Autodesk Inventor part; units mm, degrees
ref_plane "Work Plane1" through (0, 0, 99) normal (0, 0, 1) x (1, 0, 0)
ref_plane "YZ Plane" through (0, 0, 0) normal (1, 0, 0) x (0, 1, 0)
ref_plane "XZ Plane" through (0, 0, 0) normal (0, 1, 0) x (-1, 0, 0)
sketch "Sketch1" plane through (0, 0, 0) normal (0, 0, 1) x (1, 0, 0)
  circle A0 centre (0, 0) radius 33.5
  dimension "d0" = 67
extrude "Extrusion1" add sketch "Sketch1" along normal blind 89
sketch "Sketch2" plane through (0, 0, 0) normal (0, 0, -1) x (-1, 0, 0)
  circle A0 centre (0, 0) radius 14.75
  dimension "d3" = 29.5
extrude "Extrusion2" add sketch "Sketch2" along normal blind 11
fillet "Fillet1" radius 1 3 edges at (14.75, 0, -11) (-33.5, 0, 0) (-33.5, 0, 89)
sketch "Sketch3" plane through (0, 0, 89) normal (0, 0, 1) x (1, 0, 0)
  circle A0 centre (0, 0) radius 33.5
  circle A1 centre (0, 0) radius 6.75
  dimension "d7" = 13.5
extrude "Extrusion3" cut sketch "Sketch3" against normal blind 2 contours A1
sketch "Sketch4" plane through (0, 0, 87) normal (0, 0, 1) x (1, 0, 0)
  circle A0 centre (0, 0) radius 4
  dimension "d10" = 8
ref_plane "Work Plane1" through (0, 0, 99) normal (0, 0, 1) x (1, 0, 0)
extrude "Extrusion4" add sketch "Sketch4" along normal up to surface (12 mm away)
sketch "Sketch5" plane through (0, 0, 99) normal (0, 0, 1) x (1, 0, 0)
  circle A0 centre (0, 0) radius 32.5 construction
  circle A1 centre (0, 0) radius 8.5
  dimension "d14" = 17
extrude "Extrusion5" add sketch "Sketch5" along normal blind 3
sketch "Sketch6" plane through (0, 0, 102) normal (0, 0, 1) x (1, 0, 0)
  circle A0 centre (0, 0) radius 8.5
  line L0 (-2.5, 4.3301) -> (2.5, 4.3301)
  line L1 (2.5, 4.3301) -> (5, 0)
  line L2 (5, 0) -> (2.5, -4.3301)
  line L3 (2.5, -4.3301) -> (-2.5, -4.3301)
  line L4 (-2.5, -4.3301) -> (-5, 0)
  line L5 (-5, 0) -> (-2.5, 4.3301)
  line L6 (-46.9, 0) -> (46.9, 0) construction
  dimension "d17" = 10
extrude "Extrusion6" add sketch "Sketch6" along normal blind 8.33 contours L0 L1 L2 L3 L4 L5
properties part number "MY6812-12VDC-120W"
Build history of the part. All positions in model axes, mm. A direction names the side the tool comes from. Coordinates: 2 decimals unless noted, no trailing zeros. Write each loop counter-clockwise with the first axis right and the second up, starting at its lowest first coordinate (ties: lowest second). Pieces come first, ordered by that corner, then holes. Notation, with made-up numbers: (-28, 16.25) -> (9, 16.25) arc R15 cw to (9, 41.25) -> close; hole circle Ø6 at (77.5, -12). An arc over 180 degrees is marked (long way). Use CSV: the item, a comma, the result in double quotes. Start each with the question number.
Q1. Drill centre lines: probe 1 along Y at (x, z) = (0, 87.65); probe 2 along Z at (x, y) = (-28.5, -4); probe 3 along Z at (x, y) = (-5.5, -6). Where is each one in solid material? Low to high.
Q2. Cut at B-B, the plane z = 77.5. List the corners of the cut face in (x, y).
Q3. Pull direction Y, two halves, no side cores. Call faces 1 (the flat face through (0, 0, 110.33)), 2 (the cylindrical face through (-1.46, -6.59, 88.01)), 3 (the flat face through (-3.77, 2.13, 106.11)): released by +Y, released by -Y, zero draft, split by the parting line, or undercut.
Q4. 3-axis set-ups, long thin cutter, end or side, ignore diameter. For faces 4 (the cylindrical face through (4.57, -7.167, 100.479)), 5 (the flat face through (7, -14, 0)), 6 (the flat face through (4, -2, 99)): which of +Z, -Z, +X, -X, +Y, -Y reach the whole face in a straight line?
Q5. Flat gauge pins, fed straight in: pin 1 Ø2 at (x, y) = (-5.5, 18.5) entering from +Z; pin 2 Ø5.5 at (x, z) = (0, 105.5) entering from -Y; pin 3 Ø6 at (x, y) = (13.5, 12.5) entering from -Z. Where does each tip first touch, or does it go through?
Checked values:
1,probe 1,"y = -33.5 to -6.75, -4 to 4, 6.75 to 33.5"
1,probe 2,"z = 0 to 89"
1,probe 3,"z = -11 to 89, 99 to 102"
2,outline,"circle Ø67 at (0, 0)"
3,face 1,"zero draft"
3,face 2,"undercut"
3,face 3,"released by +Y"
4,face 4,"+Z"
4,face 5,"-Z"
4,face 6,"none"
5,pin 1,"stops at z = 89"
5,pin 2,"stops at y = -4.33"
5,pin 3,"stops at z = 0"
